```python
from build123d import *

# Parameters (mm, degrees)
WYCI_GNI_CIE_CIENKA_CIANKA1_DEPTH      = 400
WYCI_GNI_CIE_CIENKA_CIANKA1_DEPTH_BACK = 400
LUSTRO2_START                          = 277.039042492
LUSTRO2_DEPTH                          = 3.5
DODANIE_WYCI_GNI_CIE1_DEPTH            = 2
WYCI_GNI_CIE_CIENKA_CIANKA2_DEPTH      = 10
SZKIC12_R                              = 2.5
WYTNIJ_WYCI_GNI_CIE1_DEPTH             = 6
DODANIE_WYCI_GNI_CIE2_DEPTH            = 2
WYCI_GNI_CIE_CIENKA_CIANKA3_DEPTH      = 10
SZKIC16_R                              = 2.5
WYTNIJ_WYCI_GNI_CIE2_DEPTH             = 6
DODANIE_WYCI_GNI_CIE3_DEPTH            = 2
WYCI_GNI_CIE_CIENKA_CIANKA4_DEPTH      = 10
SZKIC19_R                              = 2.5
WYTNIJ_WYCI_GNI_CIE3_DEPTH             = 6
EXTRUDE_THIN1_START                    = 6
SZKIC19_2_R                            = 4.5
SZKIC19_2_R_2                          = 2.5
EXTRUDE_THIN1_DEPTH                    = 6
EXTRUDE_THIN2_START                    = 6
SZKIC16_2_R                            = 4.5
SZKIC16_2_R_2                          = 2.5
EXTRUDE_THIN2_DEPTH                    = 6
EXTRUDE_THIN3_START                    = 6
SZKIC12_2_R                            = 4.5
SZKIC12_2_R_2                          = 2.5
EXTRUDE_THIN3_DEPTH                    = 6


# Read off the part's stored shape, not the designer's step: Lustro2
with BuildPart() as part:
    # Szkic1 → Wyciągnięcie-cienka ścianka1 (new, two sides: drawn at the far end of the back side and taken through both)
    with BuildSketch(Plane(origin=(0, 0, 0), x_dir=(1, 0, 0), z_dir=(0, 1, 0)).offset(-WYCI_GNI_CIE_CIENKA_CIANKA1_DEPTH_BACK)):
        Polygon((972.134722106, -477.320983834), (957.040530502, -464.199803255), (959.008707589, -461.935674514), (958.253998008, -461.279615485), (545, -102.043395667), (517.881642578, -102.043395667), (517.881642578, -102.543395667), (544.81305766, -102.543395667), (957.925968494, -461.656970275), (958.303323284, -461.98499979), (956.335146197, -464.24912853), (971.806692592, -477.698338624), align=None)
    extrude(amount=WYCI_GNI_CIE_CIENKA_CIANKA1_DEPTH + WYCI_GNI_CIE_CIENKA_CIANKA1_DEPTH_BACK)

    # Cięcie powierzchnią2
    split(bisect_by=Plane(origin=(-13.122082675, 50.268990001, -11.406852442), x_dir=(0.6328754019355285, 0.32469887066665293, 0.7028793417171568), z_dir=(0.24669767629086262, -0.945066673459785, 0.21445101824972695)), keep=Keep.TOP)

    # Cięcie powierzchnią3
    split(bisect_by=Plane(origin=(-13.795060398, -53.64380516, -11.991863051), x_dir=(-0.7143770117085512, 0.3225312314146349, -0.6209984620790296), z_dir=(-0.24341741026967303, -0.9465588226635253, -0.21159952650099761)), keep=Keep.BOTTOM)

    # Cięcie powierzchnią4
    split(bisect_by=Plane(origin=(-24.349944471, -199.016868, -21.167083796), x_dir=(0.7449832908348125, -0.1600276007809854, 0.6476040946173941), z_dir=(-0.12077436340947467, -0.987112540183885, -0.10498755238005406)), keep=Keep.BOTTOM)

    # Cięcie powierzchnią5
    split(bisect_by=Plane(origin=(110.843151094, -553.888363867, 96.354481224), x_dir=(0.7294998198065532, 0.25630205312360615, 0.6341445185971655), z_dir=(0.19343361492315114, -0.9665967398893007, 0.1681492761005468)), keep=Keep.BOTTOM)

    # Lustro2 outline → Lustro2 (cut)
    with BuildSketch(Plane(origin=(0, 0, 0), x_dir=(0.754709580222771, 0, 0.6560590289905086), z_dir=(0.6560590289905085, 0, -0.754709580222771)).offset(LUSTRO2_START)):
        Polygon((909.445947287, -351.683941116), (805.20178126, -334.784202631), (993.753311489, -400), (1046.830129212, -400), (1046.830129212, -315.255256391), align=None)
    extrude(amount=LUSTRO2_DEPTH, mode=Mode.SUBTRACT)

    # Szkic10 → Dodanie-wyciągnięcie1 (add)
    with BuildSketch(Plane(origin=(184.050171811, 0, -211.725502995), x_dir=(-0.7547095802227711, 0, -0.6560590289905084), z_dir=(0.6560590289905084, 0, -0.7547095802227711))):
        Polygon((-723.785887875, -289.14803149), (-703.807733048, -288.213510375), (-704.274993606, -278.224432962), (-724.253148432, -279.158954077), align=None)
    dodanie_wyci_gni_cie1 = extrude(amount=DODANIE_WYCI_GNI_CIE1_DEPTH)

    # Szkic11 → Wyciągnięcie-cienka ścianka2 (add)
    with BuildSketch(Plane(origin=(185.362289869, 0, -213.234922155), x_dir=(-0.7547095802227721, 0, -0.6560590289905072), z_dir=(0.6560590289905072, 0, -0.7547095802227721))):
        Polygon((-723.785887875, -289.14803149), (-703.807733048, -288.213510375), (-703.901185159, -286.215694893), (-723.879339986, -287.150216008), align=None)
    wyci_gni_cie_cienka_cianka2 = extrude(amount=WYCI_GNI_CIE_CIENKA_CIANKA2_DEPTH)

    # Szkic12 → Wytnij-wyciągnięcie1 (cut)
    with BuildSketch(Plane(origin=(-8.922386764, -252.736192146, -7.756112483), x_dir=(0.9993780104898576, -0.03524800775504095, -0.0010817109755482265), z_dir=(0.035264601930747055, 0.9989077413419046, 0.030655050772765847))):
        with Locations(Location((736.803075954, -260.021158903, 0), (0, 0, 179.937993373))):
            Circle(SZKIC12_R)
    wytnij_wyci_gni_cie1 = extrude(amount=-WYTNIJ_WYCI_GNI_CIE1_DEPTH, mode=Mode.SUBTRACT)

    # Szkic14 → Dodanie-wyciągnięcie2 (add)
    with BuildSketch(Plane(origin=(184.050171811, 0, -211.725502995), x_dir=(-0.7547095802227711, 0, -0.6560590289905084), z_dir=(0.6560590289905084, 0, -0.7547095802227711))):
        Polygon((-826.154339771, -317.666675693), (-807.050007897, -311.748525334), (-810.009083077, -302.196359397), (-829.11341495, -308.114509757), align=None)
    dodanie_wyci_gni_cie2 = extrude(amount=DODANIE_WYCI_GNI_CIE2_DEPTH)

    # Szkic15 → Wyciągnięcie-cienka ścianka3 (add)
    with BuildSketch(Plane(origin=(185.362289869, 0, -213.234922155), x_dir=(-0.7547095802227656, 8.492898931658996e-15, -0.6560590289905148), z_dir=(0.6560590289905147, 9.769962616701384e-15, -0.7547095802227655))):
        Polygon((-826.154339771, -317.666675693), (-807.050007897, -311.748525334), (-807.641822933, -309.838092146), (-826.746154807, -315.756242506), align=None)
    wyci_gni_cie_cienka_cianka3 = extrude(amount=WYCI_GNI_CIE_CIENKA_CIANKA3_DEPTH)

    # Szkic16 → Wytnij-wyciągnięcie2 (cut)
    with BuildSketch(Plane(origin=(-12.723943102, -54.423656206, -11.060754992), x_dir=(0.9747442148680406, -0.21885025353139564, -0.04447788338636554), z_dir=(0.22332423867840068, 0.9552165936601662, 0.1941327989160557))):
        with Locations(Location((839.308044037, -375.023490092, 0), (0, 0, 177.401291281))):
            Circle(SZKIC16_R)
    wytnij_wyci_gni_cie2 = extrude(amount=-WYTNIJ_WYCI_GNI_CIE2_DEPTH, mode=Mode.SUBTRACT)

    # Szkic17 → Dodanie-wyciągnięcie3 (add)
    with BuildSketch(Plane(origin=(184.050171811, 0, -211.725502995), x_dir=(-0.7547095802227711, 0, -0.6560590289905084), z_dir=(0.6560590289905084, 0, -0.7547095802227711))):
        Polygon((-980.419174897, -315.823054253), (-960.869985355, -320.045516598), (-958.758754182, -310.270921827), (-978.307943724, -306.048459483), align=None)
    dodanie_wyci_gni_cie3 = extrude(amount=DODANIE_WYCI_GNI_CIE3_DEPTH)

    # Szkic18 → Wyciągnięcie-cienka ścianka4 (add)
    with BuildSketch(Plane(origin=(185.362289869, 0, -213.234922155), x_dir=(-0.7547095802227731, -3.9689825973234995e-15, -0.656059028990506), z_dir=(0.656059028990506, -4.565792188770957e-15, -0.7547095802227731))):
        Polygon((-980.419174897, -315.823054253), (-960.869985355, -320.045516598), (-960.44773912, -318.090597644), (-979.996928662, -313.868135299), align=None)
    wyci_gni_cie_cienka_cianka4 = extrude(amount=WYCI_GNI_CIE_CIENKA_CIANKA4_DEPTH)

    # Szkic19 → Wytnij-wyciągnięcie3 (cut)
    with BuildSketch(Plane(origin=(81.850178316, -502.114472254, 71.151274498), x_dir=(0.9872243085600819, 0.15776060888456483, -0.022355197884150288), z_dir=(-0.15933663918907087, 0.9774594770966201, -0.138509227295274))):
        with Locations(Location((849.886383223, -371.032714173, 0), (0, 0, 178.706565483))):
            Circle(SZKIC19_R)
    wytnij_wyci_gni_cie3 = extrude(amount=-WYTNIJ_WYCI_GNI_CIE3_DEPTH, mode=Mode.SUBTRACT)

    # Szkic19<2> → Extrude-Thin1 (add)
    with BuildSketch(Plane(origin=(81.850178316, -502.114472254, 71.151274498), x_dir=(0.9872243085600819, 0.15776060888456483, -0.022355197884150288), z_dir=(-0.15933663918907087, 0.9774594770966201, -0.138509227295274)).offset(EXTRUDE_THIN1_START)):
        with Locations((849.886383223, -371.032714173)):
            Circle(SZKIC19_2_R)
        with Locations((849.886383223, -371.032714173)):
            Circle(SZKIC19_2_R_2, mode=Mode.SUBTRACT)
    extrude_thin1 = extrude(amount=-EXTRUDE_THIN1_DEPTH)

    # Szkic16<2> → Extrude-Thin2 (add)
    with BuildSketch(Plane(origin=(-12.723943102, -54.423656206, -11.060754992), x_dir=(0.9747442148680406, -0.21885025353139564, -0.04447788338636554), z_dir=(0.22332423867840068, 0.9552165936601662, 0.1941327989160557)).offset(EXTRUDE_THIN2_START)):
        with Locations((839.308044037, -375.023490092)):
            Circle(SZKIC16_2_R)
        with Locations((839.308044037, -375.023490092)):
            Circle(SZKIC16_2_R_2, mode=Mode.SUBTRACT)
    extrude_thin2 = extrude(amount=-EXTRUDE_THIN2_DEPTH)

    # Szkic12<2> → Extrude-Thin3 (add)
    with BuildSketch(Plane(origin=(-8.922386764, -252.736192146, -7.756112483), x_dir=(0.9993780104898576, -0.03524800775504095, -0.0010817109755482265), z_dir=(0.035264601930747055, 0.9989077413419046, 0.030655050772765847)).offset(EXTRUDE_THIN3_START)):
        with Locations((736.803075954, -260.021158903)):
            Circle(SZKIC12_2_R)
        with Locations((736.803075954, -260.021158903)):
            Circle(SZKIC12_2_R_2, mode=Mode.SUBTRACT)
    extrude_thin3 = extrude(amount=-EXTRUDE_THIN3_DEPTH)

    # Lustro3: Dodanie-wyciągnięcie1, Wyciągnięcie-cienka ścianka2, Wytnij-wyciągnięcie1, Dodanie-wyciągnięcie2, Wyciągnięcie-cienka ścianka3, Wytnij-wyciągnięcie2, Dodanie-wyciągnięcie3, Wyciągnięcie-cienka ścianka4, Wytnij-wyciągnięcie3, Extrude-Thin1, Extrude-Thin2, Extrude-Thin3 across plane
    add(dodanie_wyci_gni_cie1.mirror(Plane.ZX))
    add(wyci_gni_cie_cienka_cianka2.mirror(Plane.ZX))
    add(wytnij_wyci_gni_cie1.mirror(Plane.ZX), mode=Mode.SUBTRACT)
    add(dodanie_wyci_gni_cie2.mirror(Plane.ZX))
    add(wyci_gni_cie_cienka_cianka3.mirror(Plane.ZX))
    add(wytnij_wyci_gni_cie2.mirror(Plane.ZX), mode=Mode.SUBTRACT)
    add(dodanie_wyci_gni_cie3.mirror(Plane.ZX))
    add(wyci_gni_cie_cienka_cianka4.mirror(Plane.ZX))
    add(wytnij_wyci_gni_cie3.mirror(Plane.ZX), mode=Mode.SUBTRACT)
    add(extrude_thin1.mirror(Plane.ZX))
    add(extrude_thin2.mirror(Plane.ZX))
    add(extrude_thin3.mirror(Plane.ZX))


solid = part.part
```
Model file for the job. Use its own axes, mm. A direction names the side the tool comes from. Coordinates: 2 decimals unless noted, no trailing zeros. Order: outer loops, then holes, each group sorted by start corner. A loop starts at its lowest first (then second) coordinate and runs counter-clockwise, first axis right, second up. Notation, with made-up numbers: (35.5, 15.25) -> (79.5, 15.25) arc R32 cw to (79.5, 51.25) -> close; hole circle Ø2 at (53, -12.75). An arc over 180 degrees is marked (long way). Return JSON: item names as keys, results as strings.
Item 1: Mould opens along Y. For faces 1 (the face through (801.31, -311.44, 317.14)), 2 (the face through (831.535, -343.367, 351.461)), 3 (the face through (922.284, 333.385, 430.452)) say: pulls with the +Y half, pulls with the -Y half, needs draft (parallel to the pull), parting line crosses it, or undercut.
Model answer:
{"face 1": "undercut", "face 2": "pulls with the -Y half", "face 3": "pulls with the +Y half"}
Item 2: Slice it at C-C (z = 399). Write the cut outline in (x, y).
Model answer:
{"outline": "(885.85, -346.15) -> (886.61, -346) -> (886.61, 346) -> (885.85, 346.15) -> close"}
Item 3: Slice it at A-A (y = 40.5). Write the cut outline in (x, z) (3 decimals), then the cut area to 3 significant figures.
Model answer:
{"outline": "(517.882, 102.043) -> (545, 102.043) -> (959.009, 461.936) -> (957.041, 464.2) -> (972.135, 477.321) -> (971.807, 477.698) -> (956.335, 464.249) -> (958.303, 461.985) -> (544.813, 102.543) -> (517.882, 102.543) -> close", "area": "299 mm²"}
Item 4: Pin check, flat tips, straight feed: P1, Ø21.5, axis at x = 536.5, y = 91, coming from the +Z side; P2, Ø12, axis at y = 228.5, z = 196.5, coming from the +X side; P3, Ø2, axis at x = 815, y = -150, coming from the -Z side. Stop position of each tip, or through.
Model answer:
{"P1": "stops at z = 104.66", "P2": "stops at x = 660.56", "P3": "stops at z = 335.88"}
Item 5: Slice it at B-B (x = 942.5). Write the cut outline in (y, z), then the cut area to 3 significant figures.
Model answer:
{"outline": "(-326.36, 447.58) -> (326.36, 447.58) -> (326.24, 448.25) -> (-326.24, 448.25) -> close", "area": "432 mm²"}
Item 6: 3-axis set-ups, long thin cutter, end or side, ignore diameter. For faces 4 (the face through (921.354, 317.436, 423.131)), 5 (the face through (915.555, 308.189, 422.856)), 6 (the face through (531, -4, 102.543)), 7 (the face through (805.06, -315.41, 322.04)), 8 (the face through (801.31, 311.44, 317.14)): which of +Z, -Z, +X, -X, +Y, -Y reach the whole face in a straight line?
Model answer:
{"face 4": "+X, +Y", "face 5": "-Z", "face 6": "+Z, -X, +Y, -Y", "face 7": "-Z, -Y", "face 8": "none"}
Item 7: Wall check: line 1 along Z through (x, y) = (541, 174); line 2 along Z through (x, y) = (939.5, 296); line 3 along X through (y, z) = (-61, 157). Give the ranges that are in metal, low to high. Write a range as from..to.
Model answer:
{"line 1": "z = 102.04..102.54", "line 2": "z = 444.98..445.64", "line 3": "x = 607.46..608.22"}
